Here's how the part is built. I have some questions about the finished solid (model axes, mm). Face numbers are marked on the shaded views. A direction names the side the tool comes from. Coordinates: 2 decimals unless noted, no trailing zeros. Write each loop counter-clockwise with the first axis right and the second up, starting at its lowest first coordinate (ties: lowest second). Pieces come first, ordered by that corner, then holes.
(1) Imagine slicing it at A-A, the plane x = 46. List the corners of the cut face in (y, z) for me.
(2) Imagine slicing it at D-D, the plane x = 65.5. List the corners of the cut face in (y, z) for me, plus the area to 3 significant figures.
(3) Thinking about a two-plate mould opening in Y: for the marked faces 1, 2 and 3, which applies, released by +Y, released by -Y, zero draft, split by the parting line, or undercut?
(4) Please list where these lines run through material, in increasing order: probe 1 along Y at (x, z) = (25, 4); probe 2 along X at (y, z) = (20, 1.8); probe 3 along Y at (x, z) = (64, 3.1).
(5) Which directions (+Z, -Z, +X, -X, +Y, -Y) give clear straight access to the entire face, cutting with the end or side of a thin tool? Please do the marked faces 4 and 5.
(6) Imagine slicing it at B-B, the plane y = 17.5. List the corners of the cut face in (x, z) for me, plus the area to 3 significant figures.
(7) Imagine slicing it at C-C, the plane z = 1.3. List the corners of the cut face in (x, y) for me.
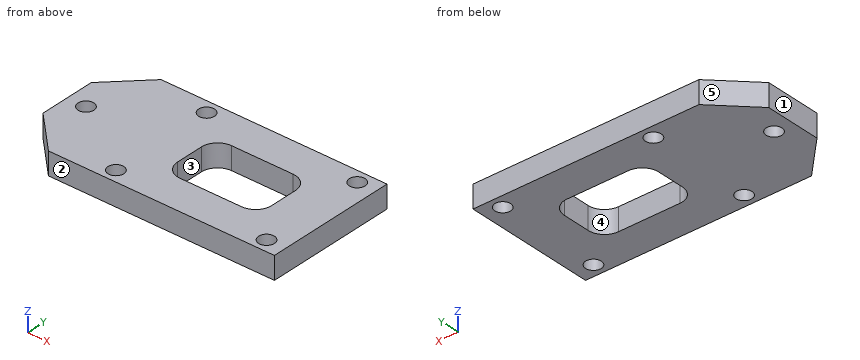
```python
from build123d import *

# Parameters (mm, degrees)
SZKIC1_R                    = 2.1
DODANIE_WYCI_GNI_CIE1_DEPTH = 6


with BuildPart() as part:
    # Szkic1 → Dodanie-wyciągnięcie1 (new body)
    with BuildSketch(Plane.XY):
        Polygon((10, 0), (70, 0), (70, 35), (10, 35), (0, 25), (0, 10), align=None)
        with Locations((65, 31.6)):
            Circle(SZKIC1_R, mode=Mode.SUBTRACT)
        with Locations((25, 31.6)):
            Circle(SZKIC1_R, mode=Mode.SUBTRACT)
        with Locations(Location((65, 3.4, 0), (0, 0, 180))):
            Circle(SZKIC1_R, mode=Mode.SUBTRACT)
        with Locations(Location((25, 3.4, 0), (0, 0, 180))):
            Circle(SZKIC1_R, mode=Mode.SUBTRACT)
        with Locations((5, 17.5)):
            Circle(SZKIC1_R, mode=Mode.SUBTRACT)
        with BuildLine():
            Line((53.188946254, 9.5), (36.811053746, 9.5))
            ThreePointArc((36.811053746, 9.5), (33.762678408, 10.762678408), (32.5, 13.811053746))
            Line((32.5, 13.811053746), (32.5, 21.188946254))
            ThreePointArc((32.5, 21.188946254), (33.762678408, 24.237321592), (36.811053746, 25.5))
            Line((36.811053746, 25.5), (53.188946254, 25.5))
            ThreePointArc((53.188946254, 25.5), (56.237321592, 24.237321592), (57.5, 21.188946254))
            Line((57.5, 21.188946254), (57.5, 13.811053746))
            ThreePointArc((57.5, 13.811053746), (56.237321592, 10.762678408), (53.188946254, 9.5))
        make_face(mode=Mode.SUBTRACT)
    extrude(amount=DODANIE_WYCI_GNI_CIE1_DEPTH)


solid = part.part
```
Recorded:
1. outline: (0, 0) - (9.5, 0) - (9.5, 6) - (0, 6) - close; (25.5, 0) - (35, 0) - (35, 6) - (25.5, 6) - close
2. outline: (0, 0) - (1.36, 0) - (1.36, 6) - (0, 6) - close; (5.44, 0) - (29.56, 0) - (29.56, 6) - (5.44, 6) - close; (33.64, 0) - (35, 0) - (35, 6) - (33.64, 6) - close
2. area: 161 mm2
3. face 1: zero draft
3. face 2: released by -Y
3. face 3: undercut
4. probe 1: y = 0 to 1.3, 5.5 to 29.5, 33.7 to 35
4. probe 2: x = 0 to 32.5, 57.5 to 70
4. probe 3: y = 0 to 1.55, 5.25 to 29.75, 33.45 to 35
5. face 4: +Z, -Z
5. face 5: +Z, -Z, -X, +Y
6. outline: (0, 0) - (2.9, 0) - (2.9, 6) - (0, 6) - close; (7.1, 0) - (32.5, 0) - (32.5, 6) - (7.1, 6) - close; (57.5, 0) - (70, 0) - (70, 6) - (57.5, 6) - close
6. area: 245 mm2
7. outline: (0, 10) - (10, 0) - (70, 0) - (70, 35) - (10, 35) - (0, 25) - close; hole circle Ø4.2 at (5, 17.5); hole circle Ø4.2 at (25, 3.4); hole circle Ø4.2 at (25, 31.6); hole (32.5, 13.81) arc R4.31 ccw to (36.81, 9.5) - (53.19, 9.5) arc R4.31 ccw to (57.5, 13.81) - (57.5, 21.19) arc R4.31 ccw to (53.19, 25.5) - (36.81, 25.5) arc R4.31 ccw to (32.5, 21.19) - close; hole circle Ø4.2 at (65, 3.4); hole circle Ø4.2 at (65, 31.6)
